Can you work these out from the model? Positions are in its coordinate system, mm. A direction names the side the tool comes from. Give positions to 0.01 mm unless a question says otherwise; leave off trailing zeros. Loops run counter-clockwise (first coordinate to the right, second up) from the corner with the lowest first, then second, coordinate; pieces in that order, holes last. Notation, with made-up numbers: M 14.25,47 L 48.25,47 A14 ccw 48.25,53 Z; hole C -27.5,-21.75 d2. An arc over 180 degrees is marked long. Use CSV: the item, a comma, the result in double quotes.
from build123d import *

# Parameters (mm, degrees)
SKETCH1_W               = 77.6
SKETCH1_H               = 61.3
BOSS_EXTRUDE1_DEPTH     = 7
SKETCH2_W               = 95.2
SKETCH2_H               = 78.9
SKETCH2_W_2             = 75.2
SKETCH2_H_2             = 58.9
CUT_EXTRUDE_THIN1_DEPTH = 1.85
SKETCH3_W               = 73.6
SKETCH3_H               = 57.3
CUT_EXTRUDE1_DEPTH      = 5
FILLET1_R               = 1
CUT_EXTRUDE3_REACH      = 51.698
SKETCH5_W               = 20.41
SKETCH5_H               = 2.7
SKETCH5_W_2             = 25.49
SKETCH6_R               = 2.5
BOSS_EXTRUDE2_DEPTH     = 21.5
SKETCH7_R               = 1.2
CUT_EXTRUDE4_DEPTH      = 5
CUT_EXTRUDE5_REACH      = 55.918
SKETCH8_R               = 1
SKETCH10_R              = 2.525
CUT_EXTRUDE6_DEPTH      = 2


with BuildPart() as part:
    # Sketch1 → Boss-Extrude1 (new body)
    with BuildSketch(Plane(origin=(0, 0, 0), x_dir=(1, 0, 0), z_dir=(0, 1, 0))):
        Rectangle(SKETCH1_W, SKETCH1_H)
    extrude(amount=BOSS_EXTRUDE1_DEPTH)

    # Sketch2 → Cut-Extrude-Thin1 (cut)
    with BuildSketch(Plane(origin=(0, 7, 0), x_dir=(1, 0, 0), z_dir=(0, 1, 0))):
        Rectangle(SKETCH2_W, SKETCH2_H)
        Rectangle(SKETCH2_W_2, SKETCH2_H_2, mode=Mode.SUBTRACT)
    extrude(amount=-CUT_EXTRUDE_THIN1_DEPTH, mode=Mode.SUBTRACT)

    # Sketch3 → Cut-Extrude1 (cut)
    with BuildSketch(Plane(origin=(0, 7, 0), x_dir=(1, 0, 0), z_dir=(0, 1, 0))):
        Rectangle(SKETCH3_W, SKETCH3_H)
    extrude(amount=-CUT_EXTRUDE1_DEPTH, mode=Mode.SUBTRACT)

    # Fillet1
    fillet1_edges = [part.edges().sort_by_distance(p)[0] for p in [
        (38.8, 2.575, 30.65),
        (-38.8, 2.575, 30.65),
        (-38.8, 2.575, -30.65),
        (38.8, 2.575, -30.65),
        (36.8, 2, 0),
        (36.8, 4.5, -28.65),
        (0, 2, 28.65),
        (36.8, 4.5, 28.65),
        (-36.8, 2, 0),
        (-36.8, 4.5, 28.65),
        (0, 2, -28.65),
        (-36.8, 4.5, -28.65),
        (0, 0, 30.65),
        (-38.8, 0, 0),
        (0, 0, -30.65),
        (38.8, 0, 0),
    ]]
    fillet(fillet1_edges, radius=FILLET1_R)

    # Sketch5 → Cut-Extrude3 (cut, up to next)
    with BuildSketch(Plane(origin=(0, 2, 0), x_dir=(1, 0, 0), z_dir=(0, 1, 0)), mode=Mode.PRIVATE) as cut_extrude3_sk1:
        with Locations((20.095, -24.3)):
            Rectangle(SKETCH5_W, SKETCH5_H)
    cut_extrude3_tool1 = extrude(cut_extrude3_sk1.sketch, amount=-CUT_EXTRUDE3_REACH, mode=Mode.PRIVATE) & part.part
    # Sketch5 → Cut-Extrude3 (cut, up to next)
    with BuildSketch(Plane(origin=(0, 2, 0), x_dir=(1, 0, 0), z_dir=(0, 1, 0)), mode=Mode.PRIVATE) as cut_extrude3_sk2:
        with Locations((-4.355, -24.3)):
            Rectangle(SKETCH5_W_2, SKETCH5_H)
    cut_extrude3_tool2 = extrude(cut_extrude3_sk2.sketch, amount=-CUT_EXTRUDE3_REACH, mode=Mode.PRIVATE) & part.part
    add(cut_extrude3_tool1.solids().sort_by_distance((20.095, 2, 24.3))[0], mode=Mode.SUBTRACT)
    add(cut_extrude3_tool2.solids().sort_by_distance((-4.355, 2, 24.3))[0], mode=Mode.SUBTRACT)

    # Sketch6 → Boss-Extrude2 (add)
    with BuildSketch(Plane(origin=(0, 2, 0), x_dir=(1, 0, 0), z_dir=(0, 1, 0))):
        with Locations(Location((31.6, 19.09, 0), (0, 0, 270))):
            Circle(SKETCH6_R)
        with Locations(Location((31.6, -8.85, 0), (0, 0, 270))):
            Circle(SKETCH6_R)
        with Locations(Location((-19.5, -24.01, 0), (0, 0, 16.260204708))):
            Circle(SKETCH6_R)
        with Locations(Location((-20.8, 24.19, 0), (0, 0, 270))):
            Circle(SKETCH6_R)
    extrude(amount=BOSS_EXTRUDE2_DEPTH)

    # Sketch7 → Cut-Extrude4 (cut)
    with BuildSketch(Plane(origin=(0, 23.5, 0), x_dir=(1, 0, 0), z_dir=(0, 1, 0))):
        with Locations(Location((31.6, 19.09, 0), (0, 0, 270))):
            Circle(SKETCH7_R)
        with Locations(Location((31.6, -8.85, 0), (0, 0, 270))):
            Circle(SKETCH7_R)
        with Locations(Location((-20.8, 24.19, 0), (0, 0, 270))):
            Circle(SKETCH7_R)
        with Locations(Location((-19.5, -24.01, 0), (0, 0, 270))):
            Circle(SKETCH7_R)
    extrude(amount=-CUT_EXTRUDE4_DEPTH, mode=Mode.SUBTRACT)

    # Sketch8 → Cut-Extrude5 (cut, up to next)
    with BuildSketch(Plane(origin=(0, 2, 0), x_dir=(1, 0, 0), z_dir=(0, 1, 0)), mode=Mode.PRIVATE) as cut_extrude5_sk1:
        with Locations(Location((-28.5, -22.95, 0), (0, 0, 270))):
            Circle(SKETCH8_R)
    cut_extrude5_tool1 = extrude(cut_extrude5_sk1.sketch, amount=-CUT_EXTRUDE5_REACH, mode=Mode.PRIVATE) & part.part
    add(cut_extrude5_tool1.solids().sort_by_distance((-28.5, 2, 22.95))[0], mode=Mode.SUBTRACT)

    # Sketch10 → Cut-Extrude6 (cut)
    with BuildSketch(Plane.XZ):
        with Locations(Location((13.89, 16.95, 0), (0, 0, 270))):
            Circle(SKETCH10_R)
        with Locations(Location((19.89, 16.95, 0), (0, 0, 270))):
            Circle(SKETCH10_R)
        with Locations(Location((25.89, 16.95, 0), (0, 0, 270))):
            Circle(SKETCH10_R)
    extrude(amount=-CUT_EXTRUDE6_DEPTH, mode=Mode.SUBTRACT)


solid = part.part
Q1. I want a section at C-C, the plane x = 19.89. Please give me the cut outline in (y, z) (3 decimals), then the cut area to 3 significant figures.
Model answer:
outline,"M 0,-29.65 A1 ccw 1,-30.65 L 5.15,-30.65 L 5.15,-29.45 L 7,-29.45 L 7,-28.65 L 3,-28.65 A1 cw 2,-27.65 L 2,14.425 L 0,14.425 Z; M 0,19.475 L 2,19.475 L 2,22.95 L 0,22.95 Z; M 0,25.65 L 2,25.65 L 2,27.65 A1 cw 3,28.65 L 7,28.65 L 7,29.45 L 5.15,29.45 L 5.15,30.65 L 1,30.65 A1 ccw 0,29.65 Z"
area,"123 mm2"
Q2. If we mould it in two halves opening along Z, with no side actions, what happens to faces 1 (the flat face through (33, 23.5, 9)), 2 (the flat face through (8.39, 1, 24)), 3 (the flat face through (-1, 3, -30.65)), 4 (the cylindrical face through (32.79, 21.04, 8.69))? For each: released by +Z, released by -Z, zero draft, split by the parting line, or undercut.
Model answer:
face 1,"zero draft"
face 2,"undercut"
face 3,"released by -Z"
face 4,"undercut"
Q3. I want a section at B-B, the plane z = 16.95. Please give me the cut outline in (x, y) (3 decimals), then the cut area to 3 significant figures.
Model answer:
outline,"M -38.8,1 A1 ccw -37.8,0 L 11.365,0 L 11.365,2 L -35.8,2 A1 cw -36.8,3 L -36.8,7 L -37.6,7 L -37.6,5.15 L -38.8,5.15 Z; M 16.415,0 L 17.365,0 L 17.365,2 L 16.415,2 Z; M 22.415,0 L 23.365,0 L 23.365,2 L 22.415,2 Z; M 28.415,0 L 37.8,0 A1 ccw 38.8,1 L 38.8,5.15 L 37.6,5.15 L 37.6,7 L 36.8,7 L 36.8,3 A1 cw 35.8,2 L 28.415,2 Z"
area,"140 mm2"
Q4. For faces 5 (the flat face through (30.3, 1, 24)), 6 (the flat face through (32, 18.5, -19)), 7 (the flat face through (-17.1, 1, 24)), 8 (the flat face through (-1, 6, -29.45)), which set-ups out of +Z, -Z, +X, -X, +Y, -Y let a thin tool reach every point of the face, with its end or its side?
Model answer:
face 5,"+Y, -Y"
face 6,"+Y"
face 7,"-Y"
face 8,"-Z, +X, -X, +Y"
Q5. I want a section at D-D, the plane z = -7. Please give me the cut outline in (x, y).
Model answer:
outline,"M -38.8,1 A1 ccw -37.8,0 L 37.8,0 A1 ccw 38.8,1 L 38.8,5.15 L 37.6,5.15 L 37.6,7 L 36.8,7 L 36.8,3 A1 cw 35.8,2 L -35.8,2 A1 cw -36.8,3 L -36.8,7 L -37.6,7 L -37.6,5.15 L -38.8,5.15 Z"
Q6. Please list where these lines run through material, in increasing order: L1, parallel to X at y = 1.25, z = 16.95 (3 decimals); L2, parallel to X at y = 21.5, z = 24.01; L3, parallel to Z at x = 5, y = 6.25. Write a range as from..to.
Model answer:
L1,"-38.8..11.365, 16.415..17.365, 22.415..23.365, 28.415..38.8"
L2,"-22..-20.7, -18.3..-17"
L3,"-29.45..-28.65, 28.65..29.45"
Q7. I'm going to push flat-ended pins straight in: P1, Ø0.9, axis at x = 13, y = 6, coming from the +Z side; P2, Ø6.5, axis at x = 13.89, z = 16.95, coming from the +Y side. Where does each tip first touch, or does it pass through?
Model answer:
P1,"z = 29.45"
P2,"y = 2"
Q8. I want a section at A-A, the plane x = -12. Please give me the cut outline in (y, z).
Model answer:
outline,"M 0,-29.65 A1 ccw 1,-30.65 L 5.15,-30.65 L 5.15,-29.45 L 7,-29.45 L 7,-28.65 L 3,-28.65 A1 cw 2,-27.65 L 2,22.95 L 0,22.95 Z; M 0,25.65 L 2,25.65 L 2,27.65 A1 cw 3,28.65 L 7,28.65 L 7,29.45 L 5.15,29.45 L 5.15,30.65 L 1,30.65 A1 ccw 0,29.65 Z"
